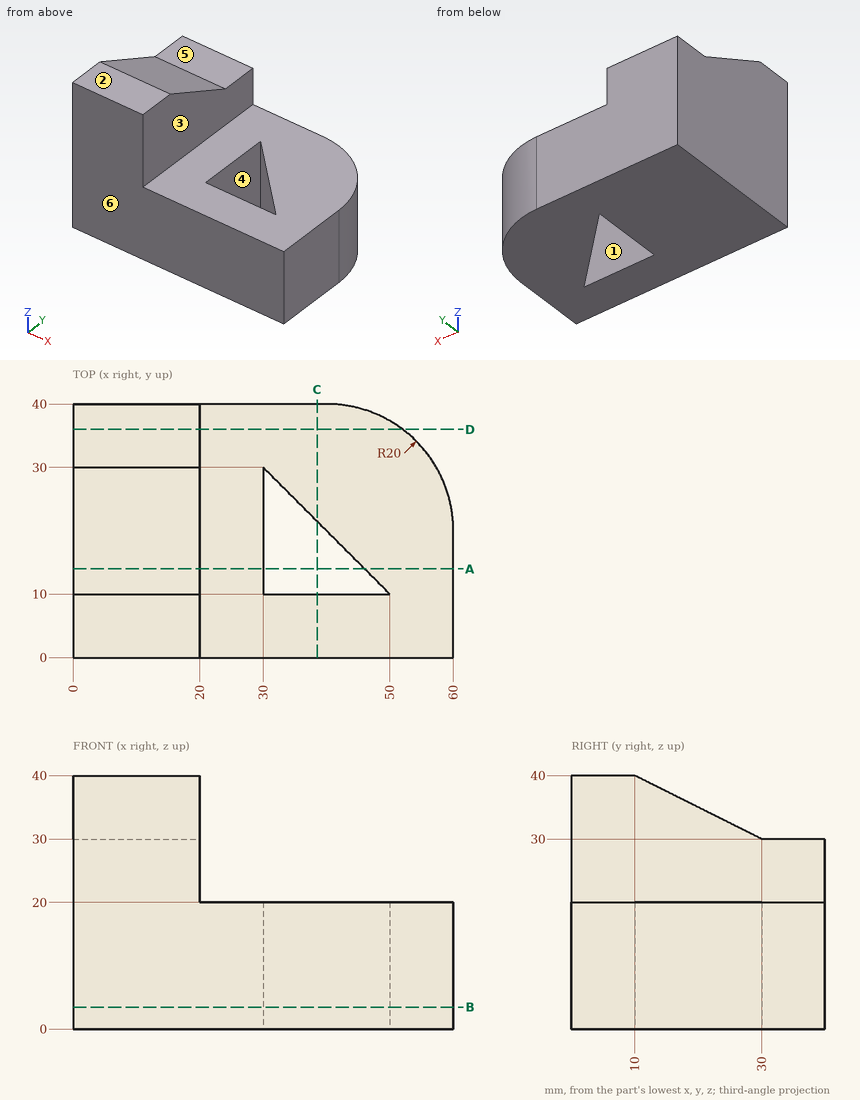
Design review of the part shown in the three views and the two pictorial views. Dimensions are in mm from the part's minimum x, y and z. A direction names the side the tool comes from. Give positions to 0.01 mm unless a question says otherwise; leave off trailing zeros. Loops run counter-clockwise (first coordinate to the right, second up) from the corner with the lowest first, then second, coordinate; pieces in that order, holes last. Notation, with made-up numbers: (-24.75, 32.25) -> (-1.75, 32.25) arc R15 cw to (-1.75, 56.25) -> close; hole circle Ø1 at (84, 55.5). An arc over 180 degrees is marked (long way). Write each question's results on one line, items separated by ' | '.
Q1. Take a section at A-A, the plane y = 14. Write out the cut boundary in (x, z), plus the area to 3 significant figures.
Reply:
outline: (0, 0) -> (30, 0) -> (30, 20) -> (20, 20) -> (20, 38) -> (0, 38) -> close; (46, 0) -> (60, 0) -> (60, 20) -> (46, 20) -> close | area: 1,240 mm²
Q2. Take a section at B-B, the plane z = 3.5. Write out the cut boundary in (x, y), plus the area to 3 significant figures.
Reply:
outline: (0, 0) -> (60, 0) -> (60, 20) arc R20 ccw to (40, 40) -> (0, 40) -> close; hole (30, 10) -> (50, 10) -> (30, 30) -> close | area: 2,110 mm²
Q3. Machinability: for the marked faces 1, 2 and 3, which of the approach directions +Z, -Z, +X, -X, +Y, -Y give a long, thin tool a straight path to every point of the face, cutting with its end or side? Answer none if there is none.
Reply:
face 1: +Z, -Z | face 2: +Z, +X, -X, +Y, -Y | face 3: +Z, +X, +Y, -Y
Q4. Wall thickness on L1, parallel to Z at x = 46, y = 20; L2, parallel to X at y = 13, z = 8.5: over which ranges is each line inside the solid? List them lowest first.
Reply:
L1: z = 0 to 20 | L2: x = 0 to 30, 47 to 60
Q5. Take a section at D-D, the plane y = 36. Write out the cut boundary in (x, z), plus the area to 3 significant figures.
Reply:
outline: (0, 0) -> (52, 0) -> (52, 20) -> (20, 20) -> (20, 30) -> (0, 30) -> close | area: 1,240 mm²
Q6. For pin 1 Ø3 at (x, y) = (13.5, 35.5) entering from +Z; pin 2 Ø8 at (y, z) = (34.5, 23.5) entering from +X; pin 3 Ø10 at (y, z) = (32.5, 16) entering from +X, all flat-tipped, find the tip position at first contact; note any pin that passes through.
Reply:
pin 1: stops at z = 30 | pin 2: stops at x = 55.56 | pin 3: stops at x = 58.54
Q7. Take a section at C-C, the plane x = 38.5. Write out the cut boundary in (y, z).
Reply:
outline: (0, 0) -> (10, 0) -> (10, 20) -> (0, 20) -> close; (21.5, 0) -> (40, 0) -> (40, 20) -> (21.5, 20) -> close
Q8. The part is to be moulded in two halves that separate along Y. For the marked faces 4, 5 and 6, say which applies: +Y half, -Y half, draft (parallel to the pull), parting line (faces both ways), or undercut.
Reply:
face 4: undercut | face 5: draft | face 6: -Y half
